```python
from build123d import *

# Parameters (mm, degrees)
F0_W     = 38.1
F0_H     = 38.1
F1_DEPTH = 19.05
F0_R     = 4.569596
F2_DEPTH = 6.35
F3_R     = 6.35
F4_DEPTH = 38.101


with BuildPart() as f1:
    # F0 (on Top) → F1 (new body, symmetric)
    with BuildSketch(Plane.XY):
        Rectangle(F0_W, F0_H)
    extrude(amount=F1_DEPTH, both=True)

    # F0 (on Top) → F2 (join, symmetric)
    with BuildSketch(Plane.XY):
        with BuildLine():
            Line((19.05, 19.05), (19.05, -19.05))
            Line((19.05, -19.05), (50.8, -19.05))
            ThreePointArc((50.8, -19.05), (69.85, 0), (50.8, 19.05))
            Line((50.8, 19.05), (19.05, 19.05))
        make_face()
        with Locations((31.75, -6.35)):
            Circle(F0_R, mode=Mode.SUBTRACT)
        with Locations((50.8, -6.35)):
            Circle(F0_R, mode=Mode.SUBTRACT)
        with Locations((31.75, 6.35)):
            Circle(F0_R, mode=Mode.SUBTRACT)
        with Locations((50.8, 6.35)):
            Circle(F0_R, mode=Mode.SUBTRACT)
    extrude(amount=F2_DEPTH, both=True)

    # F3 (on face) → F4 (cut, through all)
    with BuildSketch(Plane.XY.offset(19.05)):
        Circle(F3_R)
    extrude(amount=-F4_DEPTH, mode=Mode.SUBTRACT)


solid = f1.part
```
Part model, mm, in its own coordinate system. A direction names the side the tool comes from. Round coordinates to 2 decimals unless told otherwise and drop trailing zeros. Write each loop counter-clockwise with the first axis right and the second up, starting at its lowest first coordinate (ties: lowest second). Pieces come first, ordered by that corner, then holes. Notation, with made-up numbers: M 65.25,11 L 74.25,11 A30 cw 74.25,42 Z; hole C 81,74 d5. An arc over 180 degrees is marked long. One line per question, with ' | ' between items.
(1) Saw through at A-A on x = 31.75. Write the cut outline in (y, z).
Answer key:
outline: M -19.05,-6.35 L -10.92,-6.35 L -10.92,6.35 L -19.05,6.35 Z; M -1.78,-6.35 L 1.78,-6.35 L 1.78,6.35 L -1.78,6.35 Z; M 10.92,-6.35 L 19.05,-6.35 L 19.05,6.35 L 10.92,6.35 Z
(2) Two-plate mould, pull along X, no slides. Class faces 1 (the face through (-1.38, -6.2, 0.27)), 2 (the face through (-5, 5, -19.05)), 3 (the face through (69.845, -0.419, 0.089)): released by +X, released by -X, zero draft, split by the parting line, or undercut.
Answer key:
face 1: undercut | face 2: zero draft | face 3: released by +X
(3) 3-axis set-ups, long thin cutter, end or side, ignore diameter. For faces 4 (the face through (44, 0, -6.35)), 5 (the face through (44, 0, 6.35)), 6 (the face through (36.11, -4.98, -0.09)): which of +Z, -Z, +X, -X, +Y, -Y reach the whole face in a straight line?
Answer key:
face 4: -Z, +X, +Y, -Y | face 5: +Z, +X, +Y, -Y | face 6: +Z, -Z
(4) Pin check, flat tips, straight feed: pin 1 (1 mm diameter, centred on x = 49, y = 9, fed in from -Z); pin 2 (6.5 mm diameter, centred on y = 2, z = -12, fed in from +X); pin 3 (10.5 mm diameter, centred on x = 50.8, y = 6.35, fed in from +Z). Stop position of each tip, or through.
Answer key:
pin 1: passes through | pin 2: stops at x = 19.05 | pin 3: stops at z = 6.35
(5) Saw through at C-C on z = 5. Write the cut outline in (x, y), then the cut area to 3 significant figures.
Answer key:
outline: M -19.05,-19.05 L 50.8,-19.05 A19.05 ccw 50.8,19.05 L -19.05,19.05 Z; hole C 0,0 d12.7; hole C 31.75,-6.35 d9.14; hole C 31.75,6.35 d9.14; hole C 50.8,-6.35 d9.14; hole C 50.8,6.35 d9.14 | area: 2,840 mm^2
(6) Probe line 1 along Y through (x, z) = (50.8, 2.5); line 2 along X through (y, z) = (-5, 5.5); line 3 along Y through (x, z) = (29.5, 5.5). List the from-to ranges inside material, lowest first.
Answer key:
line 1: y = -19.05 to -10.92, -1.78 to 1.78, 10.92 to 19.05 | line 2: x = -19.05 to -3.91, 3.91 to 27.38, 36.12 to 46.43, 55.17 to 69.18 | line 3: y = -19.05 to -10.33, -2.37 to 2.37, 10.33 to 19.05
(7) Saw through at B-B on y = 0. Write the cut outline in (x, z).
Answer key:
outline: M -19.05,-19.05 L -6.35,-19.05 L -6.35,19.05 L -19.05,19.05 Z; M 6.35,-19.05 L 19.05,-19.05 L 19.05,-6.35 L 69.85,-6.35 L 69.85,6.35 L 19.05,6.35 L 19.05,19.05 L 6.35,19.05 Z
(8) Saw through at D-D on x = 0. Write the cut outline in (y, z), then the cut area to 3 significant figures.
Answer key:
outline: M -19.05,-19.05 L -6.35,-19.05 L -6.35,19.05 L -19.05,19.05 Z; M 6.35,-19.05 L 19.05,-19.05 L 19.05,19.05 L 6.35,19.05 Z | area: 968 mm^2
